The model under review builds one solid part; all positions refer to its coordinate system, in mm. A direction names the side the tool comes from. Give positions to 0.01 mm unless a question says otherwise; leave off trailing zeros. Order: outer loops, then holes, each group sorted by start corner. A loop starts at its lowest first (then second) coordinate and runs counter-clockwise, first axis right, second up. Notation, with made-up numbers: (62.25, 17.5) - (111.25, 17.5) arc R16 cw to (111.25, 33.5) - close; hole circle Ø4 at (-2, -39). An arc over 180 degrees is marked (long way). Use CSV: the item, a comma, the result in double quotes. Start each with the question number.
1. For pin 1 (2 mm diameter, centred on y = -71, z = -4.5, fed in from -X); pin 2 (2 mm diameter, centred on y = -187, z = -3.5, fed in from +X), all flat-tipped, find the tip position at first contact; note any pin that passes through.
2. Take a section at A-A, the plane x = 0. State the section outline as (y, z) points, then the cut area to 3 significant figures.
3. Take a section at B-B, the plane z = 0. State the section outline as (x, y) points, then the cut area to 3 significant figures.
4. Take a section at C-C, the plane y = 32.5. State the section outline as (x, z) points, then the cut area to 3 significant figures.
5. Machinability: for faces 1 (the flat face through (-1.42, 230, 3.92)), 2 (the cylindrical face through (-0.867, -227.182, -3.905)), 3 (the cylindrical face through (-6, 11, 0)), which of the approach directions +Z, -Z, +X, -X, +Y, -Y give a long, thin tool a straight path to every point of the face, cutting with its end or side? Answer none if there is none.
6. To check wall thickness, follow line 1 (Y direction, x = -2.25, z = 4); line 2 (X direction, y = 161.5, z = -0.25); line 3 (X direction, y = -172.5, z = 4.5). State the ranges of each line that lie inside material, in increasing order. Write a range as [from, to].
```python
from build123d import *

# Parameters (mm, degrees)
SKETCH1_R           = 6
BOSS_EXTRUDE1_DEPTH = 240
SKETCH2_R           = 6
SKETCH2_R_2         = 4
CUT_EXTRUDE1_DEPTH  = 10
SKETCH3_R           = 6
SKETCH3_R_2         = 4
CUT_EXTRUDE2_DEPTH  = 25.999999878


with BuildPart() as part:
    # Sketch1 → Boss-Extrude1 (new body, symmetric)
    with BuildSketch(Plane(origin=(0, 0, 0), x_dir=(1, 0, 0), z_dir=(0, 1, 0))):
        Circle(SKETCH1_R)
    extrude(amount=BOSS_EXTRUDE1_DEPTH, both=True)

    # Sketch2 → Cut-Extrude1 (cut)
    with BuildSketch(Plane(origin=(0, 240, 0), x_dir=(1, 0, 0), z_dir=(0, 1, 0))):
        Circle(SKETCH2_R)
        Circle(SKETCH2_R_2, mode=Mode.SUBTRACT)
    extrude(amount=-CUT_EXTRUDE1_DEPTH, mode=Mode.SUBTRACT)

    # Sketch3 → Cut-Extrude2 (cut)
    with BuildSketch(Plane.XZ.offset(240)):
        Circle(SKETCH3_R)
        Circle(SKETCH3_R_2, mode=Mode.SUBTRACT)
    extrude(amount=-CUT_EXTRUDE2_DEPTH, mode=Mode.SUBTRACT)


solid = part.part
```
Determined:
1,pin 1,"stops at x = -4.87"
1,pin 2,"stops at x = 5.45"
2,outline,"(-240, -4) - (-214, -4) - (-214, -6) - (230, -6) - (230, -4) - (240, -4) - (240, 4) - (230, 4) - (230, 6) - (-214, 6) - (-214, 4) - (-240, 4) - close"
2,area,"5,620 mm²"
3,outline,"(-6, -214) - (-4, -214) - (-4, -240) - (4, -240) - (4, -214) - (6, -214) - (6, 230) - (4, 230) - (4, 240) - (-4, 240) - (-4, 230) - (-6, 230) - close"
3,area,"5,620 mm²"
4,outline,"circle Ø12 at (0, 0)"
4,area,"113 mm²"
5,face 1,"+Y"
5,face 2,"-Y"
5,face 3,"+Y, -Y"
6,line 1,"y = [-214, 230]"
6,line 2,"x = [-5.99, 5.99]"
6,line 3,"x = [-3.97, 3.97]"
